Design review of the part built by this model. Coordinates are the model's own, in mm. Coordinates: 2 decimals unless noted, no trailing zeros. Loops run counter-clockwise (first coordinate to the right, second up) from the corner with the lowest first, then second, coordinate; pieces in that order, holes last.
Q1. Wall thickness on probe 1 along Z at (x, y) = (0.55, -1.75); probe 2 along Z at (x, y) = (0.35, -0.75); probe 3 along Y at (x, z) = (0.6, 43): over which ranges is each line inside the solid? List them lowest first.
Q2. Draft analysis for pull direction Z (two halves, no side actions). For faces 1 (the face through (0.493, -2.423, 1.567)), 2 (the face through (1, 0, 44)), state which applies: released by +Z, released by -Z, zero draft, split by the parting line, or undercut.
Q3. Add section A-A on x = 0.4. Give the boundary of the cut face in (y, z).
```python
from build123d import *

# Parameters (mm, degrees)
SKETCH_1_W      = 120
SKETCH_1_H      = 10
SKETCH_1_R      = 1.5
EXTRUDE_1_DEPTH = 1


with BuildPart() as part:
    # 草图1 → 凸台-拉伸1 (new body)
    with BuildSketch(Plane(origin=(0, 0, 0), x_dir=(0, 0, -1), z_dir=(1, 0, 0))):
        with Locations((-42.952312312, -1.848982316)):
            Rectangle(SKETCH_1_W, SKETCH_1_H)
        with Locations((-82.952312312, -1.848982316)):
            Circle(SKETCH_1_R, mode=Mode.SUBTRACT)
        with Locations((-2.952312312, -1.848982316)):
            Circle(SKETCH_1_R, mode=Mode.SUBTRACT)
        with Locations((-92.952312312, -1.848982316)):
            Circle(SKETCH_1_R, mode=Mode.SUBTRACT)
        with Locations((7.047687688, -1.848982316)):
            Circle(SKETCH_1_R, mode=Mode.SUBTRACT)
        with Locations((-42.952312312, -1.848982316)):
            Circle(SKETCH_1_R, mode=Mode.SUBTRACT)
    extrude(amount=EXTRUDE_1_DEPTH)


solid = part.part
```
Entries:
1. probe 1: z = -17.05 to -8.54, -5.55 to 1.46, 4.45 to 41.46, 44.45 to 81.46, 84.45 to 91.46, 94.45 to 102.95
1. probe 2: z = -17.05 to -8.07, -6.03 to 1.93, 3.97 to 41.93, 43.97 to 81.93, 83.97 to 91.93, 93.97 to 102.95
1. probe 3: y = -6.85 to -3.35, -0.35 to 3.15
2. face 1: undercut
2. face 2: zero draft
3. outline: (-6.85, -17.05) - (3.15, -17.05) - (3.15, 102.95) - (-6.85, 102.95) - close; hole circle Ø3 at (-1.85, -7.05); hole circle Ø3 at (-1.85, 2.95); hole circle Ø3 at (-1.85, 42.95); hole circle Ø3 at (-1.85, 82.95); hole circle Ø3 at (-1.85, 92.95)
